Check sheet for the modelled part. Datum: model origin and axes. Units: mm. A direction names the side the tool comes from. Give positions to 0.01 mm unless a question says otherwise; leave off trailing zeros. Loops run counter-clockwise (first coordinate to the right, second up) from the corner with the lowest first, then second, coordinate; pieces in that order, holes last.
```python
from build123d import *

# Parameters (mm, degrees)
PAD005_DEPTH    = 30
PAD006_DEPTH    = 30
SKETCH043_R     = 0.9
POCKET016_DEPTH = 5


with BuildPart() as part:
    # Sketch037 → Pad005 (new body)
    with BuildSketch(Plane.XZ.offset(-45)):
        with BuildLine():
            ThreePointArc((-10.178404, -6.708561), (-5.503497, -7.075491), (-1.569892, -4.522816))
            ThreePointArc((1.569892, -4.522816), (0, -3.761944), (-1.569892, -4.522816))
            ThreePointArc((1.569892, -4.522816), (5.503497, -7.075491), (10.178405, -6.708561))
            ThreePointArc((10.875556, -7.168051), (10.650715, -6.750573), (10.178405, -6.708561))
            Line((10.875556, -12), (10.875556, -7.168051))
            Line((10.875556, -12), (-10.875555, -12))
            Line((-10.875555, -12), (-10.875555, -7.168051))
            ThreePointArc((-10.178404, -6.708561), (-10.650714, -6.750574), (-10.875555, -7.168051))
        make_face()
    extrude(amount=PAD005_DEPTH)

    # Sketch042 → Pad006 (join)
    with BuildSketch(Plane.XZ.offset(-45)):
        Polygon((-4, -12), (0, -16), (4, -12), align=None)
    extrude(amount=PAD006_DEPTH)

    # Sketch043 → Pocket016 (cut)
    with BuildSketch(Plane.XY.offset(-9)):
        with Locations((-5.5, 30)):
            Circle(SKETCH043_R)
        with Locations((-5.5, -30)):
            Circle(SKETCH043_R)
        with Locations((5.5, 30)):
            Circle(SKETCH043_R)
        with Locations((5.5, -30)):
            Circle(SKETCH043_R)
    extrude(amount=-POCKET016_DEPTH, mode=Mode.SUBTRACT)


solid = part.part
```
(1) Section check A-A on x = -5. Record the boundary of the cut face in (y, z).
(2) Gauge pin test, flat ends, axial feed: pin 1 Ø5 at (y, z) = (28.5, -5.5) entering from +X; pin 2 Ø8 at (x, y) = (5, 31) entering from -Z; pin 3 Ø1.4 at (x, y) = (6, 30.5) entering from -Z; pin 4 Ø1.5 at (x, y) = (-6.5, 33.5) entering from +Z. Record the tip position at first contact, or that the pin passes through.
(3) Access from +Z, -Z, +X, -X, +Y, -Y to the whole of each face (thin tool, end or side, straight path). Record for faces 4 (the face through (-6.4, 30, -10.5)), 5 (the face through (7, 30, -12)), 6 (the face through (10.876, 30, -10)).
(4) Material ranges on line 1 (Y direction, x = -5.5, z = -9.95); line 2 (Z direction, x = -7.5, y = 34.5); line 3 (X direction, y = 23.5, z = -13.5), recorded low to high.
(5) Section check B-B on z = -13. Record the boundary of the cut face in (x, y), plus the area to 3 significant figures.
(6) Section check D-D on y = 37.75. Record the boundary of the cut face in (x, z), plus the area to 3 significant figures.
(7) Section check C-C on y = 30. Record the boundary of the cut face in (x, z), plus the area to 3 significant figures.
(8) Release check for a two-part mould opening along X. For faces 1 (the face through (4.6, 30, -10.5)), 2 (the face through (-7, 30, -12)), 3 (the face through (-10.876, 30, -10)) record: pulls with the +X half, pulls with the -X half, needs draft (parallel to the pull), parting line crosses it, or undercut.
Computed values:
1. outline: (15, -12) - (29.25, -12) - (29.25, -9) - (30.75, -9) - (30.75, -12) - (45, -12) - (45, -6.93) - (15, -6.93) - close
2. pin 1: stops at x = 10.88
2. pin 2: stops at z = -15
2. pin 3: stops at z = -12
2. pin 4: stops at z = -7.13
3. face 4: -Z
3. face 5: -Z, +X, +Y, -Y
3. face 6: +Z, -Z, +X, +Y, -Y
4. line 1: y = 15 to 29.1, 30.9 to 45
4. line 2: z = -12 to -7.3
4. line 3: x = -2.5 to 2.5
5. outline: (-3, 15) - (3, 15) - (3, 45) - (-3, 45) - close
5. area: 180 mm2
6. outline: (-10.88, -12) - (-4, -12) - (0, -16) - (4, -12) - (10.88, -12) - (10.88, -7.17) arc R0.5 ccw to (10.18, -6.71) arc R7.3 cw to (1.57, -4.52) arc R2 ccw to (-1.57, -4.52) arc R7.3 cw to (-10.18, -6.71) arc R0.5 ccw to (-10.88, -7.17) - close
6. area: 140 mm2
7. outline: (-10.88, -12) - (-6.4, -12) - (-6.4, -9) - (-4.6, -9) - (-4.6, -12) - (-4, -12) - (0, -16) - (4, -12) - (4.6, -12) - (4.6, -9) - (6.4, -9) - (6.4, -12) - (10.88, -12) - (10.88, -7.17) arc R0.5 ccw to (10.18, -6.71) arc R7.3 cw to (1.57, -4.52) arc R2 ccw to (-1.57, -4.52) arc R7.3 cw to (-10.18, -6.71) arc R0.5 ccw to (-10.88, -7.17) - close
7. area: 129 mm2
8. face 1: undercut
8. face 2: needs draft
8. face 3: pulls with the -X half
